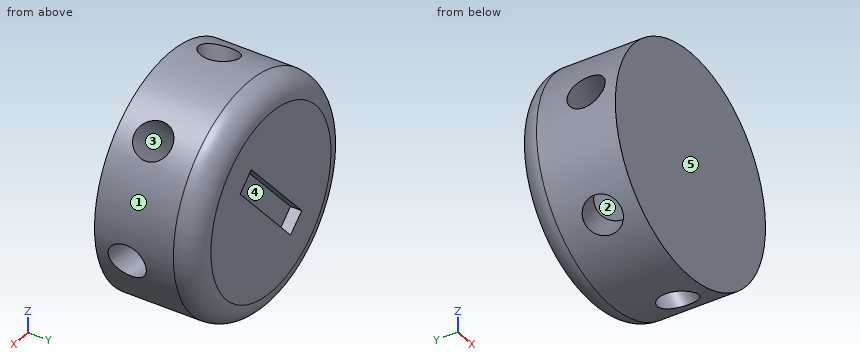
from build123d import *

# Parameters (mm, degrees)
BASE_DEPTH         = 3
BASE_DEPTH_BACK    = 6
SKETCH1_R          = 10
SKETCH2_R          = 1.6
HOLE1_DEPTH        = 19.646604683
HOLE1MIRROR_COUNT  = 2
SKETCH3_R          = 1.6
HOLE2_DEPTH        = 19.158121362
HOLE2MIRROR_COUNT  = 2
SKETCH4_R          = 1.6
HOLE3_DEPTH        = 19.100993715
HOLE3MIRROR_COUNT  = 2
FILLET1_R          = 2
CUT_EXTRUDE1_DEPTH = 1


with BuildPart() as part:
    # Sketch1 → base (new, two sides: drawn at the far end of the back side and taken through both)
    with BuildSketch(Plane(origin=(0, 0, 0), x_dir=(1, 0, 0), z_dir=(0, 1, 0)).offset(-BASE_DEPTH_BACK)):
        with Locations(Location((0, 0, 0), (0, 0, 270))):
            Circle(SKETCH1_R)
    extrude(amount=BASE_DEPTH + BASE_DEPTH_BACK)

    # Sketch2 → hole1 (cut, through all)
    with BuildSketch(Plane(origin=(2.670502563, -1.093066116, 2.770130417), x_dir=(-0.6558691872850446, 0.22429081675253856, 0.7207837669443827), z_dir=(-0.6676256406563905, 0.27326652891267483, -0.692532604369038))):
        with Locations(Location((0, 0, 0), (0, 0, 346.516491398))):
            Circle(SKETCH2_R)
    hole1 = extrude(amount=-HOLE1_DEPTH, mode=Mode.SUBTRACT)

    # hole1mirror: hole1 ×2 about axis
    hole1mirror_axis = Axis((0, 5.5, 0), (0, -1, 0))
    for i in range(1, HOLE1MIRROR_COUNT):
        add(hole1.rotate(hole1mirror_axis, i * 360 / HOLE1MIRROR_COUNT), mode=Mode.SUBTRACT)

    # Sketch3 → hole2 (cut, through all)
    with BuildSketch(Plane(origin=(-0.941672921, -1.236067977, 3.685836142), x_dir=(-0.9718935871364875, 0.07382318789513377, -0.22354639834264944), z_dir=(0.23541823021467095, 0.3090169943749464, -0.921459035481267))):
        with Locations(Location((0, 0, 0), (0, 0, 90.062171088))):
            Circle(SKETCH3_R)
    hole2 = extrude(amount=-HOLE2_DEPTH, mode=Mode.SUBTRACT)

    # hole2mirror: hole2 ×2 about axis
    hole2mirror_axis = Axis((0, 5.5, 0), (0, -1, 0))
    for i in range(1, HOLE2MIRROR_COUNT):
        add(hole2.rotate(hole2mirror_axis, i * 360 / HOLE2MIRROR_COUNT), mode=Mode.SUBTRACT)

    # Sketch4 → hole3 (cut, through all)
    with BuildSketch(Plane(origin=(-3.717841, -1.236067977, 0.806098168), x_dir=(-0.19123247894507908, -0.06357892752956036, -0.979483465389136), z_dir=(0.9294602499075393, 0.30901699437494623, -0.20152454200243008))):
        with Locations(Location((0, 0, 0), (0, 0, 90))):
            Circle(SKETCH4_R)
    hole3 = extrude(amount=-HOLE3_DEPTH, mode=Mode.SUBTRACT)

    # hole3mirror: hole3 ×2 about axis
    hole3mirror_axis = Axis((0, 5.5, 0), (0, -1, 0))
    for i in range(1, HOLE3MIRROR_COUNT):
        add(hole3.rotate(hole3mirror_axis, i * 360 / HOLE3MIRROR_COUNT), mode=Mode.SUBTRACT)

    # Fillet1
    fillet1_edges = [part.edges().sort_by_distance(p)[0] for p in [
        (0, 3, -10),
    ]]
    fillet(fillet1_edges, radius=FILLET1_R)

    # Sketch6 → Cut-Extrude1 (cut)
    with BuildSketch(Plane(origin=(0, 3, 0), x_dir=(1, 0, 0), z_dir=(0, 1, 0))):
        Polygon((-4.100143947, 3.031306586), (-2.61886111, 4.375107597), (4.100143947, -3.031306586), (2.61886111, -4.375107597), align=None)
    extrude(amount=-CUT_EXTRUDE1_DEPTH, mode=Mode.SUBTRACT)


solid = part.part
Can you work these out from the model? Positions are in its coordinate system, mm. Face numbers are marked on the shaded views. A direction names the side the tool comes from. Coordinates: 2 decimals unless noted, no trailing zeros. Loops run counter-clockwise (first coordinate to the right, second up) from the corner with the lowest first, then second, coordinate; pieces in that order, holes last. Notation, with made-up numbers: M 18.25,53.25 L 59.25,53.25 A31 cw 59.25,84.25 Z; hole C -20.75,87.25 d9. An arc over 180 degrees is marked long. Answer as CSV lines item,"result". Start each with the question number.
1. Suppose I cut it at A-A, the plane y = 0.75. List the corners of the cut face in (x, z) for me, plus the area to 3 significant figures.
2. Suppose I cut it at B-B, the plane z = 0. Count the separate pieces of the cut face and the enclosed holes in it, plus the area to 3 significant figures.
3. For pin 1 Ø2 at (x, y) = (-4.5, -4.5) entering from +Z; pin 2 Ø5 at (x, y) = (7, -2.5) entering from -Z, each with a flat end and sliding along its axis, tell me the tip position at first contact or that it passes through.
4. Thinking about a two-plate mould opening in Y: for the marked faces 3, 4 and 5, which applies, +Y half, -Y half, draft (parallel to the pull), parting line (faces both ways), or undercut?
5. If I drill on probe 1 along X at (y, z) = (-2.75, 5.25); probe 2 along Z at (x, y) = (-5.5, -2.25); probe 3 along X at (y, z) = (-1.25, -6.5), over which ranges is the centre line in solid material (lowest first)? Write a range as [from, to].
6. For the marked faces 1 and 2, which set-ups out of +Z, -Z, +X, -X, +Y, -Y let a thin tool reach every point of the face, with its end or its side?
Output:
1,outline,"C 0,0 d20"
1,area,"314 mm^2"
2,separate pieces,"1"
2,enclosed holes,"2"
2,area,"161 mm^2"
3,pin 1,"stops at z = 9.37"
3,pin 2,"stops at z = -8.93"
4,face 3,"undercut"
4,face 4,"+Y half"
4,face 5,"-Y half"
5,probe 1,"x = [-8.51, -2.75], [-0.08, 3.31], [7.26, 8.51]"
5,probe 2,"z = [-8.35, -7.92], [-3.49, -0.36], [2.8, 8.35]"
5,probe 3,"x = [-7.6, -7.22], [-4.45, 0.22], [2.96, 7.6]"
6,face 1,"+Y, -Y"
6,face 2,"none"
